from build123d import *

# Parameters (mm, degrees)
F0_R     = 5
F1_DEPTH = 8
F2_W     = 20
F2_H     = 25
F2_R     = 5
F3_DEPTH = 4.9


with BuildPart() as f1:
    # F0 (on Top) → F1 (new body)
    with BuildSketch(Plane.XY):
        Polygon((-5, -12.5), (20, -12.5), (20, 12.5), (-5, 12.5), (-7.729777, 5), (-7.729777, -5), align=None)
        with Locations((10, 0)):
            Circle(F0_R, mode=Mode.SUBTRACT)
    extrude(amount=F1_DEPTH)

    # F2 (on Top) → F3 (join)
    with BuildSketch(Plane.XY):
        with Locations((10, 0)):
            Rectangle(F2_W, F2_H)
        with Locations((10, 0)):
            Circle(F2_R, mode=Mode.SUBTRACT)
    extrude(amount=-F3_DEPTH)


solid = f1.part
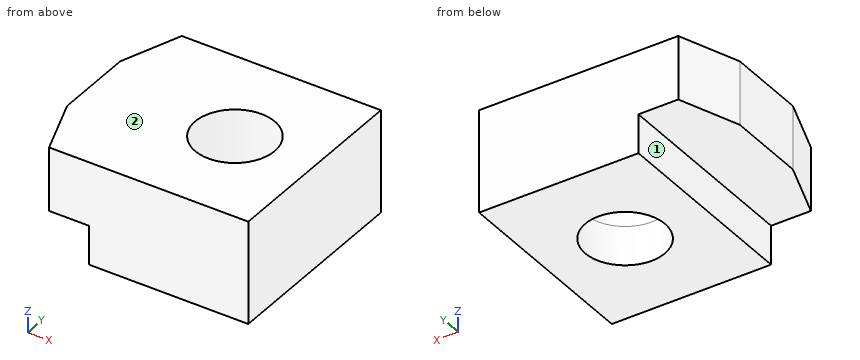
Could you check a few things on this model? Use its own coordinates, in mm. Face numbers are marked on the shaded views. A direction names the side the tool comes from. Give positions to 0.01 mm unless a question says otherwise; leave off trailing zeros. Order: outer loops, then holes, each group sorted by start corner. A loop starts at its lowest first (then second) coordinate and runs counter-clockwise, first axis right, second up.
1. I need wall thicknesses on L1, parallel to X at y = 0.25, z = 4.75; L2, parallel to Y at x = 10, z = 2.5; L3, parallel to Z at x = -4, y = -2.5. Which ranges of each line are inside material? Lowest first, please.
2. Suppose I cut it at D-D (y = 8.5). List the corners of the cut face in (x, z) for me.
3. Will these pins go through, and if not, where does the flat tip stop? P1, Ø3, axis at y = 8, z = 3.5, coming from the -X side; P2, Ø2.5, axis at x = -2.5, y = 3, coming from the -Z side.
4. Suppose I cut it at A-A (y = 0). List the corners of the cut face in (x, z) for me.
5. Suppose I cut it at C-C (z = 5.5). List the corners of the cut face in (x, y) for me.
6. For the marked faces 1 and 2, which set-ups out of +Z, -Z, +X, -X, +Y, -Y let a thin tool reach every point of the face, with its end or its side?
7. Suppose I cut it at B-B (x = 10). List the corners of the cut face in (y, z) for me, plus the area to 4 significant figures.
Solved:
1. L1: x = -7.73 to 5.01, 14.99 to 20
1. L2: y = -12.5 to -5, 5 to 12.5
1. L3: z = 0 to 8
2. outline: (-6.46, 0) - (0, 0) - (0, -4.9) - (20, -4.9) - (20, 8) - (-6.46, 8) - close
3. P1: stops at x = -7.18
3. P2: stops at z = 0
4. outline: (-7.73, 0) - (0, 0) - (0, -4.9) - (5, -4.9) - (5, 8) - (-7.73, 8) - close; (15, -4.9) - (20, -4.9) - (20, 8) - (15, 8) - close
5. outline: (-7.73, -5) - (-5, -12.5) - (20, -12.5) - (20, 12.5) - (-5, 12.5) - (-7.73, 5) - close; hole circle Ø10 at (10, 0)
6. face 1: -Z, -X, +Y, -Y
6. face 2: +Z, +X, -X, +Y, -Y
7. outline: (-12.5, -4.9) - (-5, -4.9) - (-5, 8) - (-12.5, 8) - close; (5, -4.9) - (12.5, -4.9) - (12.5, 8) - (5, 8) - close
7. area: 193.5 mm2
